Input: dimensioned drawing with shaded views. Units: mm. Origin: part minimum x, y, z. Coordinates: 2 decimals unless noted, no trailing zeros. Order: outer loops, then holes, each group sorted by start corner. A loop starts at its lowest first (then second) coordinate and runs counter-clockwise, first axis right, second up. Notation, with made-up numbers: (37, 11.5) - (81, 11.5) arc R30 ccw to (81, 43.5) - close; hole circle Ø5 at (-34.75, -23.75). An arc over 180 degrees is marked (long way). Answer as CSV lines item,"result". Start each with the question number.
Item 1: First-contact query: pin 1 (4 mm diameter, centred on x = 20, y = 18.5, fed in from +Z) (1 decimal); pin 2 (8 mm diameter, centred on y = 12, z = 24, fed in from +X); pin 3 (15 mm diameter, centred on y = 10, z = 24, fed in from +X) (1 decimal). Flat tips, straight axial feed; report the tip coordinate or a pass-through.
Item 2: Section D-D (z = 24.5). Output: boundary loops of the cut face in (x, y).
Item 3: Section C-C (x = 33). Output: boundary loops of the cut face in (y, z) (1 decimal).
Item 4: Section A-A (z = 17). Output: boundary loops of the cut face in (x, y), and give its area (3 significant figures).
Item 5: Material intervals for line 1 along X through (y, z) = (14.5, 24.5) (1 decimal); line 2 along X through (y, z) = (12, 13); line 3 along Z through (x, y) = (22, 13.25) (1 decimal), sorted ascending.
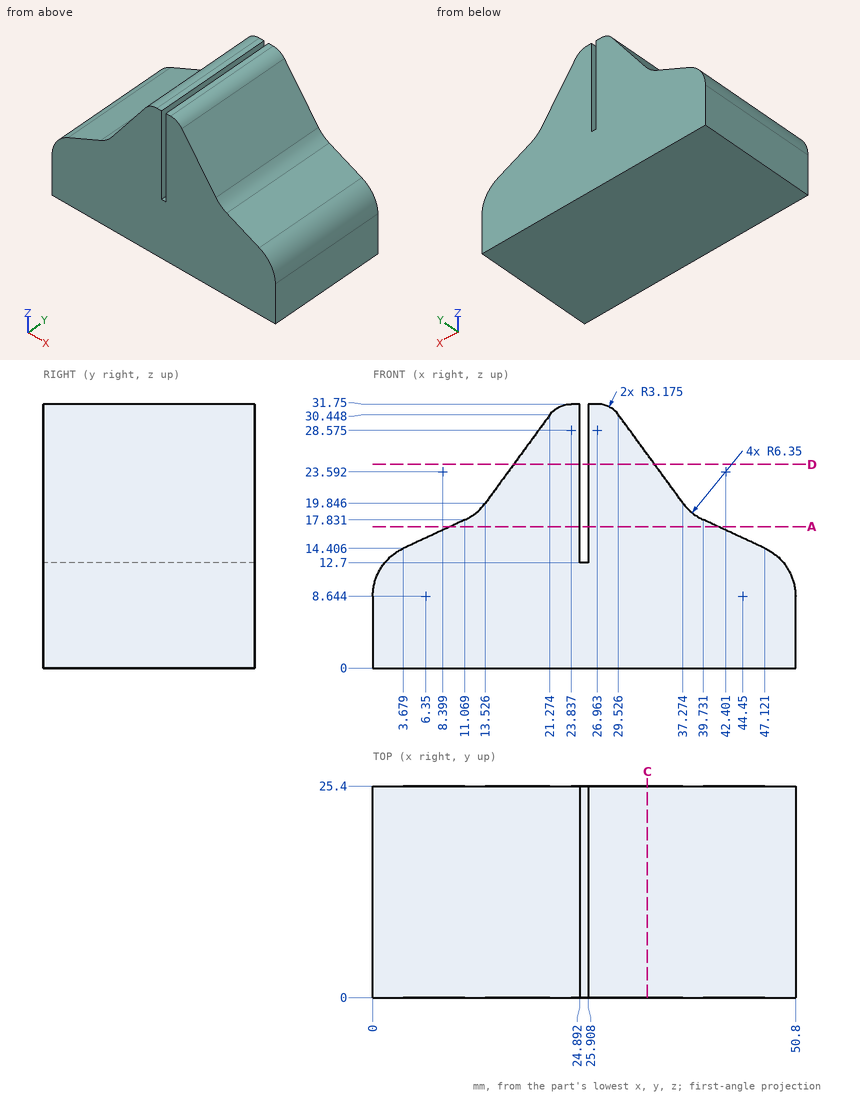
Determined:
1,pin 1,"stops at z = 31.2"
1,pin 2,"stops at x = 37.16"
1,pin 3,"stops at x = 42.6"
2,outline,"(16.93, 0) - (24.89, 0) - (24.89, 25.4) - (16.93, 25.4) - close; (25.91, 0) - (33.87, 0) - (33.87, 25.4) - (25.91, 25.4) - close"
3,outline,"(0, 0) - (25.4, 0) - (25.4, 25.7) - (0, 25.7) - close"
4,outline,"(9.28, 0) - (24.89, 0) - (24.89, 25.4) - (9.28, 25.4) - close; (25.91, 0) - (41.52, 0) - (41.52, 25.4) - (25.91, 25.4) - close"
4,area,"793 mm^2"
5,line 1,"x = 16.9 to 24.9, 25.9 to 33.9"
5,line 2,"x = 1.73 to 24.89, 25.91 to 49.07"
5,line 3,"z = 0 to 31.2"
